```python
from build123d import *

# Parameters (mm, degrees)
BOSS_EXTRUDE1_DEPTH = 20
SKETCH2_R           = 43.5
CUT_EXTRUDE2_DEPTH  = 81.006249756
SKETCH3_R           = 45
CUT_EXTRUDE3_DEPTH  = 8


with BuildPart() as part:
    # Sketch1 → Boss-Extrude1 (new body)
    with BuildSketch(Plane(origin=(0, 0, 0), x_dir=(1, 0, 0), z_dir=(0, 1, 0))):
        with BuildLine():
            Line((-49, -34.626579386), (-49, 34.626579386))
            ThreePointArc((-49, 34.626579386), (0, 60), (49, 34.626579386))
            Line((49, 34.626579386), (49, -34.626579386))
            ThreePointArc((49, -34.626579386), (0, -60), (-49, -34.626579386))
        make_face()
    extrude(amount=BOSS_EXTRUDE1_DEPTH)

    # Sketch2 → Cut-Extrude2 (cut, through all)
    with BuildSketch(Plane.XZ):
        with Locations(Location((0, 0, 0), (0, 0, 270))):
            Circle(SKETCH2_R)
    extrude(amount=-CUT_EXTRUDE2_DEPTH, mode=Mode.SUBTRACT)

    # Sketch3 → Cut-Extrude3 (cut)
    with BuildSketch(Plane(origin=(0, 20, 0), x_dir=(1, 0, 0), z_dir=(0, 1, 0))):
        with Locations(Location((0, 0, 0), (0, 0, 270))):
            Circle(SKETCH3_R)
    extrude(amount=-CUT_EXTRUDE3_DEPTH, mode=Mode.SUBTRACT)


solid = part.part
```
Geometry: final body of the model. Coordinates: model frame, mm. A direction names the side the tool comes from. Round coordinates to 2 decimals unless told otherwise and drop trailing zeros. Order: outer loops, then holes, each group sorted by start corner. A loop starts at its lowest first (then second) coordinate and runs counter-clockwise, first axis right, second up. Notation, with made-up numbers: (8, 41.25) - (52, 41.25) arc R6 ccw to (52, 48.25) - close; hole circle Ø11 at (39.25, 34.5). An arc over 180 degrees is marked (long way). Write item = value, one per line. Start each with the question number.
Q1. Cut plane A-A on x = 0. Return the cut outline in (y, z), and give its area (3 significant figures).
Q2. Pull-direction query (Z, two-part tool) for faces 1 (the cylindrical face through (-17.235, 16.056, 41.569)), 2 (the cylindrical face through (0.803, 9.86, 59.995)), 3 (the flat face through (44, 0, -1)); classes: +Z half, -Z half, draft (parallel to the pull), parting line (faces both ways), or undercut.
Q3. Cut plane D-D on y = 1.25. Return the cut outline in (x, z), and give its area (3 significant figures).
Q4. Cut plane B-B on z = 0. Return the cut outline in (x, y), and give its area (3 significant figures).
Q5. Ray query, line 1 (X direction, y = 9.5, z = 0); line 2 (X direction, y = 16.5, z = 0); line 3 (Z direction, x = -18.5, y = 14.75). Return the intervals inside material, ascending. Write a range as from..to.
Q6. Access query for faces 4 (the flat face through (22, 20, -40)), 5 (the flat face through (24, 12, -37)). Directions: +Z, -Z, +X, -X, +Y, -Y. A direction counts if a zero-diameter tool reaches every point of the face in a straight line with its end or side. Return the directions, or none.
Q7. Cut plane C-C on y = 18. Return the cut outline in (x, z).
Q8. Pin query (flat end, axial travel): pin 1 (6 mm diameter, centred on y = 13, z = 44, fed in from -X); pin 2 (5 mm diameter, centred on x = -17, y = 16.5, fed in from -Z); pin 3 (1.5 mm diameter, centred on x = -7, y = 6.5, fed in from +Z). Return the tip coordinate at first contact, or that it passes through.
Outcome:
q1.outline = (0, -60) - (20, -60) - (20, -45) - (12, -45) - (12, -43.5) - (0, -43.5) - close; (0, 43.5) - (12, 43.5) - (12, 45) - (20, 45) - (20, 60) - (0, 60) - close
q1.area = 636 mm^2
q2.face_1 = undercut
q2.face_2 = +Z half
q2.face_3 = draft
q3.outline = (-49, -34.63) arc R60 ccw to (49, -34.63) - (49, 34.63) arc R60 ccw to (-49, 34.63) - close; hole circle Ø87 at (0, 0)
q3.area = 4,330 mm^2
q4.outline = (-49, 0) - (-43.5, 0) - (-43.5, 12) - (-45, 12) - (-45, 20) - (-49, 20) - close; (43.5, 0) - (49, 0) - (49, 20) - (45, 20) - (45, 12) - (43.5, 12) - close
q4.area = 196 mm^2
q5.line_1 = -49..-43.5, 43.5..49
q5.line_2 = -49..-45, 45..49
q5.line_3 = -57.08..-41.02, 41.02..57.08
q6.face_4 = +Z, -Z, +X, -X, +Y
q6.face_5 = +Y
q7.outline = (-49, -34.63) arc R60 ccw to (49, -34.63) - (49, 34.63) arc R60 ccw to (-49, 34.63) - close; hole circle Ø90 at (0, 0)
q8.pin_1 = -43.81
q8.pin_2 = -58.22
q8.pin_3 = 59.67
